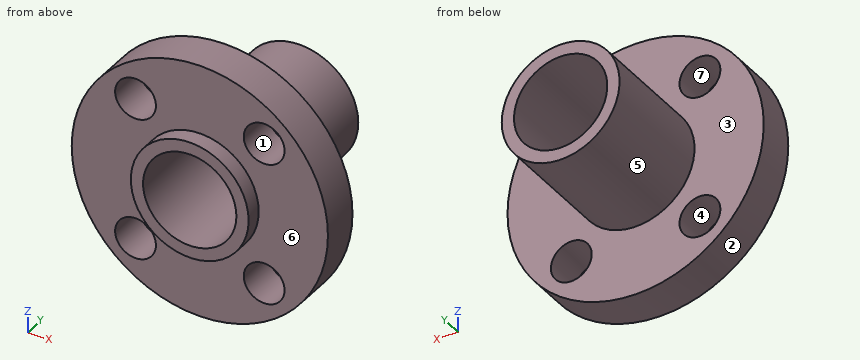
```python
from build123d import *

# Parameters (mm, degrees)
CROQUIS2_R              = 10.98
CROQUIS2_R_2            = 1.75
SALIENTE_EXTRUIR1_DEPTH = 3.36
CROQUIS3_R              = 5.05
SALIENTE_EXTRUIR2_DEPTH = 10.26
CROQUIS4_R              = 5.05
SALIENTE_EXTRUIR3_DEPTH = 1.38
CROQUIS5_R              = 4
CORTAR_EXTRUIR1_DEPTH   = 16


with BuildPart() as part:
    # Croquis2 → Saliente-Extruir1 (new body)
    with BuildSketch(Plane(origin=(0, 0, 0), x_dir=(1, 0, 0), z_dir=(0, 1, 0))):
        Circle(CROQUIS2_R)
        with Locations((-5.512093558, 6.111442105)):
            Circle(CROQUIS2_R_2, mode=Mode.SUBTRACT)
        with Locations((-5.512093558, -6.111442105)):
            Circle(CROQUIS2_R_2, mode=Mode.SUBTRACT)
        with Locations((5.512093558, -6.111442105)):
            Circle(CROQUIS2_R_2, mode=Mode.SUBTRACT)
        with Locations((5.512093558, 6.111442105)):
            Circle(CROQUIS2_R_2, mode=Mode.SUBTRACT)
    extrude(amount=SALIENTE_EXTRUIR1_DEPTH)

    # Croquis3 → Saliente-Extruir2 (add)
    with BuildSketch(Plane(origin=(0, 3.36, 0), x_dir=(1, 0, 0), z_dir=(0, 1, 0))):
        Circle(CROQUIS3_R)
    extrude(amount=SALIENTE_EXTRUIR2_DEPTH)

    # Croquis4 → Saliente-Extruir3 (add)
    with BuildSketch(Plane.XZ):
        Circle(CROQUIS4_R)
    extrude(amount=SALIENTE_EXTRUIR3_DEPTH)

    # Croquis5 → Cortar-Extruir1 (cut, through all)
    with BuildSketch(Plane(origin=(0, 13.62, 0), x_dir=(1, 0, 0), z_dir=(0, 1, 0))):
        Circle(CROQUIS5_R)
    extrude(amount=-CORTAR_EXTRUIR1_DEPTH, mode=Mode.SUBTRACT)


solid = part.part
```
Geometry check sheet. Reference: the model listing, model coordinates, mm. Face numbers are marked on the shaded views. A direction names the side the tool comes from. Give positions to 0.01 mm unless a question says otherwise; leave off trailing zeros. Loops run counter-clockwise (first coordinate to the right, second up) from the corner with the lowest first, then second, coordinate; pieces in that order, holes last. Notation, with made-up numbers: M -8,-38 L 38,-38 A10 cw 38,-31 Z; hole C -27,68.5 d6. An arc over 180 degrees is marked long. Answer as CSV lines item,"result".
Item 1: Cross-section at A-A on z = 0. Record the cut outline in (x, y).
Values:
outline,"M -10.98,0 L -5.05,0 L -5.05,-1.38 L -4,-1.38 L -4,13.62 L -5.05,13.62 L -5.05,3.36 L -10.98,3.36 Z; M 4,-1.38 L 5.05,-1.38 L 5.05,0 L 10.98,0 L 10.98,3.36 L 5.05,3.36 L 5.05,13.62 L 4,13.62 Z"
Item 2: Release check for a two-part mould opening along Z. For the marked faces 1, 2, 3 and 4 record: pulls with the +Z half, pulls with the -Z half, needs draft (parallel to the pull), parting line crosses it, or undercut.
Values:
face 1,"undercut"
face 2,"parting line crosses it"
face 3,"needs draft"
face 4,"undercut"
Item 3: Cross-section at C-C on x = 6.25. Record the cut outline in (y, z).
Values:
outline,"M 0,-9.03 L 3.36,-9.03 L 3.36,-7.7 L 0,-7.7 Z; M 0,-4.52 L 3.36,-4.52 L 3.36,4.52 L 0,4.52 Z; M 0,7.7 L 3.36,7.7 L 3.36,9.03 L 0,9.03 Z"
Item 4: Cross-section at B-B on x = 0. Record the cut outline in (y, z).
Values:
outline,"M -1.38,-5.05 L 0,-5.05 L 0,-10.98 L 3.36,-10.98 L 3.36,-5.05 L 13.62,-5.05 L 13.62,-4 L -1.38,-4 Z; M -1.38,4 L 13.62,4 L 13.62,5.05 L 3.36,5.05 L 3.36,10.98 L 0,10.98 L 0,5.05 L -1.38,5.05 Z"
Item 5: Cross-section at D-D on z = 6.5. Record the cut outline in (x, y).
Values:
outline,"M -8.85,0 L -7.22,0 L -7.22,3.36 L -8.85,3.36 Z; M -3.81,0 L 3.81,0 L 3.81,3.36 L -3.81,3.36 Z; M 7.22,0 L 8.85,0 L 8.85,3.36 L 7.22,3.36 Z"
Item 6: Material ranges on line 1 (Z direction, x = 0, y = 3.5); line 2 (X direction, y = 2.5, z = 7); line 3 (Z direction, x = 4.75, y = 2.25), recorded low to high.
Values:
line 1,"z = -5.05 to -4, 4 to 5.05"
line 2,"x = -8.46 to -7.02, -4 to 4, 7.02 to 8.46"
line 3,"z = -9.9 to -7.69, -4.54 to 4.54, 7.69 to 9.9"
Item 7: Access from +Z, -Z, +X, -X, +Y, -Y to the whole of each face (thin tool, end or side, straight path). Record for the marked faces 5, 6 and 7.
Values:
face 5,"+Y"
face 6,"-Y"
face 7,"+Y, -Y"
Item 8: Depth check by flat-ended pin: P1, Ø8, axis at x = 1, z = 8.5, coming from the +Y side; P2, Ø4, axis at x = -5.51, z = -6.11, coming from the +Y side; P3, Ø8, axis at y = 10, z = -8, coming from the +X side; P4, Ø4, axis at x = 1, y = 5.5, coming from the -Z side. Enter the tip coordinate at first touch or a pass-through.
Values:
P1,"stops at y = 13.62"
P2,"stops at y = 3.36"
P3,"stops at x = 3.08"
P4,"stops at z = -5.05"
